Source: CAD feature listing. Evaluate the final solid. Frame: model axes, mm. Face numbers are marked on the shaded views. A direction names the side the tool comes from. Give positions to 0.01 mm unless a question says otherwise; leave off trailing zeros. Loops run counter-clockwise (first coordinate to the right, second up) from the corner with the lowest first, then second, coordinate; pieces in that order, holes last. Notation, with made-up numbers: (76, -1) - (90, -1) arc R22 ccw to (90, 16) - close; hole circle Ø4 at (20.25, -11.75). An arc over 180 degrees is marked (long way). Put each result on its own line as item: value.
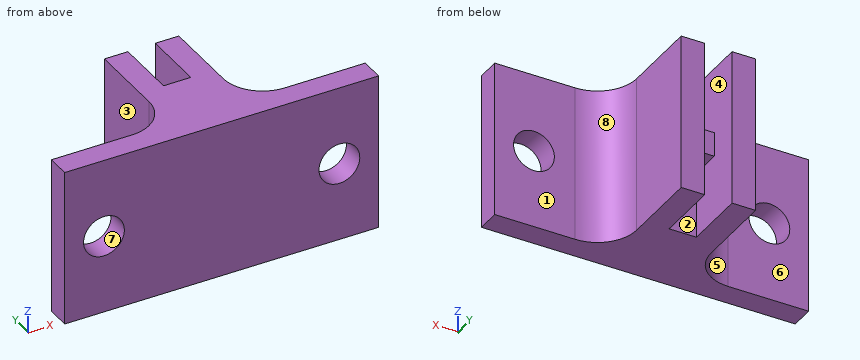
```python
from build123d import *

# Parameters (mm, degrees)
SKETCH3_W           = 40
SKETCH3_H           = 20
SKETCH3_R           = 2.6
JIG_BASE_DEPTH      = 3
SKETCH4_W           = 3
SKETCH4_H           = 20
JIG_WALL_DEPTH      = 15
STRINGER_LOCK_DEPTH = 9.48
BASE_FILET_R        = 5


with BuildPart() as part:
    # Sketch3 → Jig base (new body)
    with BuildSketch(Plane(origin=(0, 0, 0), x_dir=(1, 0, 0), z_dir=(0, 1, 0))):
        Rectangle(SKETCH3_W, SKETCH3_H)
        with Locations(Location((-15, 0, 0), (0, 0, 270))):
            Circle(SKETCH3_R, mode=Mode.SUBTRACT)
        with Locations(Location((15, 0, 0), (0, 0, 90))):
            Circle(SKETCH3_R, mode=Mode.SUBTRACT)
    extrude(amount=JIG_BASE_DEPTH)

    # Sketch4 → jig wall (add)
    with BuildSketch(Plane(origin=(0, 3, 0), x_dir=(1, 0, 0), z_dir=(0, 1, 0))):
        with Locations((-3.24, 0)):
            Rectangle(SKETCH4_W, SKETCH4_H)
        with Locations((3.24, 0)):
            Rectangle(SKETCH4_W, SKETCH4_H)
    extrude(amount=JIG_WALL_DEPTH)

    # Sketch5 → stringer lock (add)
    with BuildSketch(Plane(origin=(4.74, 0, 0), x_dir=(0, 0, -1), z_dir=(1, 0, 0))):
        Polygon((-10, 0), (10, 0), (10, 10), (1.55, 10), (1.55, 14), (-1.55, 14), (-1.55, 10), (-10, 10), align=None)
    extrude(amount=-STRINGER_LOCK_DEPTH)

    # base filet
    base_filet_edges = [part.edges().sort_by_distance(p)[0] for p in [
        (-4.74, 3, 0),
        (4.74, 3, 0),
    ]]
    fillet(base_filet_edges, radius=BASE_FILET_R)


solid = part.part
```
1) Access query for the marked faces 1, 2, 3 and 4. Directions: +Z, -Z, +X, -X, +Y, -Y. A direction counts if a zero-diameter tool reaches every point of the face in a straight line with its end or side. Return the directions, or none.
Check result:
face 1: +Z, -Z, +X, +Y
face 2: -Z, +Y
face 3: +Z, -Z, -X, +Y
face 4: +Y
2) Section query A-A, the plane x = -16. Output: boundary loops of the cut face in (y, z), plus the area to 3 significant figures.
Check result:
outline: (0, -10) - (3, -10) - (3, -2.4) - (0, -2.4) - close; (0, 2.4) - (3, 2.4) - (3, 10) - (0, 10) - close
area: 45.6 mm²
3) Material intervals for line 1 along X through (y, z) = (1.7, 0); line 2 along Z through (x, y) = (15, 2.15); line 3 along X through (y, z) = (14.5, -6), sorted ascending. Write a range as [from, to].
Check result:
line 1: [-20, -17.6], [-12.4, 12.4], [17.6, 20]
line 2: [-10, -2.6], [2.6, 10]
line 3: [-4.74, -1.74], [1.74, 4.74]
4) Section query B-B, the plane z = 0. Output: boundary loops of the cut face in (x, y), plus the area to 3 significant figures.
Check result:
outline: (-20, 0) - (-17.6, 0) - (-17.6, 3) - (-20, 3) - close; (-12.4, 0) - (12.4, 0) - (12.4, 3) - (9.74, 3) arc R5 cw to (4.74, 8) - (4.74, 18) - (1.74, 18) - (1.74, 14) - (-1.74, 14) - (-1.74, 18) - (-4.74, 18) - (-4.74, 8) arc R5 cw to (-9.74, 3) - (-12.4, 3) - close; (17.6, 0) - (20, 0) - (20, 3) - (17.6, 3) - close
area: 228 mm²
5) Section query D-D, the plane z = 5.5. Output: boundary loops of the cut face in (x, y), plus the area to 3 significant figures.
Check result:
outline: (-20, 0) - (20, 0) - (20, 3) - (9.74, 3) arc R5 cw to (4.74, 8) - (4.74, 18) - (1.74, 18) - (1.74, 10) - (-1.74, 10) - (-1.74, 18) - (-4.74, 18) - (-4.74, 8) arc R5 cw to (-9.74, 3) - (-20, 3) - close
area: 245 mm²
6) Mould query, pull axis X, two halves, no side actions, for the marked faces 5, 6, 7 and 8. Classes: pulls with the +X half, pulls with the -X half, needs draft (parallel to the pull), parting line crosses it, or undercut.
Check result:
face 5: pulls with the -X half
face 6: needs draft
face 7: undercut
face 8: pulls with the +X half
7) Pin query (flat end, axial travel): P1, Ø1.5, axis at x = -13, z = -7.5, coming from the +Y side; P2, Ø5, axis at y = 10.5, z = -2, coming from the -X side; P3, Ø1, axis at y = 15, z = -8, coming from the +X side; P4, Ø4, axis at x = 0, z = -5.5, coming from the +Y side. Return the tip coordinate at first contact, or that it passes through.
Check result:
P1: y = 3
P2: x = -4.74
P3: x = 4.74
P4: y = 18
8) Section query C-C, the plane y = 15.25. Output: boundary loops of the cut face in (x, z), plus the area to 3 significant figures.
Check result:
outline: (-4.74, -10) - (-1.74, -10) - (-1.74, 10) - (-4.74, 10) - close; (1.74, -10) - (4.74, -10) - (4.74, 10) - (1.74, 10) - close
area: 120 mm²
